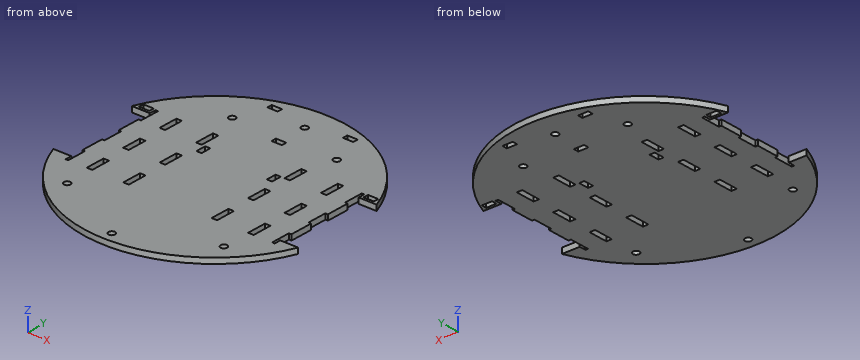
```python
from build123d import *

# Parameters (mm, degrees)
SKETCH1_R            = 127
BODY_DEPTH           = 5.334
SKETCH7_W            = 50.8
SKETCH7_H            = 88.9
WHEELCUTS_DEPTH      = 180.684310823
SKETCH4_W            = 2.4638
SKETCH4_H            = 19.05
SKETCH4_W_2          = 5.334
MOTORMOUNTS_DEPTH    = 175.099537782
SKETCH5_R            = 3.175
CASTOR_DEPTH         = 175.099537782
SKETCH6_R            = 3.175
BOLTHOLES_DEPTH      = 175.099537782
SKETCH3_W            = 10.000000066
SKETCH3_H            = 4.999999906
SKETCH3_W_2          = 5
SKETCH3_H_2          = 10
TAPESENSCUTOUT_DEPTH = 175.099537782


with BuildPart() as part:
    # Sketch1 → Body (new body)
    with BuildSketch(Plane.XY):
        Circle(SKETCH1_R)
    extrude(amount=BODY_DEPTH)

    # Sketch7 → WheelCuts (cut, through all)
    with BuildSketch(Plane.XY.offset(5.334)):
        with Locations((-127, 0)):
            Rectangle(SKETCH7_W, SKETCH7_H)
        with Locations((127, 0)):
            Rectangle(SKETCH7_W, SKETCH7_H)
    extrude(amount=-WHEELCUTS_DEPTH, mode=Mode.SUBTRACT)

    # Sketch4 → MotorMounts (cut, through all)
    with BuildSketch(Plane.XY.offset(5.334)):
        with Locations((-100.3681, 41.275)):
            Rectangle(SKETCH4_W, SKETCH4_H)
        with Locations((-100.3681, -41.275)):
            Rectangle(SKETCH4_W, SKETCH4_H)
        with Locations((-100.3681, 0)):
            Rectangle(SKETCH4_W, SKETCH4_H)
        with Locations((-78.469199932, -41.275)):
            Rectangle(SKETCH4_W_2, SKETCH4_H)
        with Locations((-78.469199932, 41.275)):
            Rectangle(SKETCH4_W_2, SKETCH4_H)
        with Locations((-78.469199932, 0)):
            Rectangle(SKETCH4_W_2, SKETCH4_H)
        with Locations((-42.966999918, -41.275)):
            Rectangle(SKETCH4_W_2, SKETCH4_H)
        with Locations((-42.966999918, 41.275)):
            Rectangle(SKETCH4_W_2, SKETCH4_H)
        with Locations((-42.966999918, 0)):
            Rectangle(SKETCH4_W_2, SKETCH4_H)
        with Locations((42.966999918, -41.275)):
            Rectangle(SKETCH4_W_2, SKETCH4_H)
        with Locations((42.966999918, 0)):
            Rectangle(SKETCH4_W_2, SKETCH4_H)
        with Locations((42.966999918, 41.275)):
            Rectangle(SKETCH4_W_2, SKETCH4_H)
        with Locations((78.469199932, -41.275)):
            Rectangle(SKETCH4_W_2, SKETCH4_H)
        with Locations((78.469199932, 0)):
            Rectangle(SKETCH4_W_2, SKETCH4_H)
        with Locations((78.469199932, 41.275)):
            Rectangle(SKETCH4_W_2, SKETCH4_H)
        with Locations((100.3681, -41.275)):
            Rectangle(SKETCH4_W, SKETCH4_H)
        with Locations((100.3681, 0)):
            Rectangle(SKETCH4_W, SKETCH4_H)
        with Locations((100.3681, 41.275)):
            Rectangle(SKETCH4_W, SKETCH4_H)
    extrude(amount=-MOTORMOUNTS_DEPTH, mode=Mode.SUBTRACT)

    # Sketch5 → Castor (cut, through all)
    with BuildSketch(Plane.XY.offset(5.334)):
        with Locations((0, -116.84)):
            Circle(SKETCH5_R)
        with Locations((0, 101.6)):
            Circle(SKETCH5_R)
    extrude(amount=-CASTOR_DEPTH, mode=Mode.SUBTRACT)

    # Sketch6 → BoltHoles (cut, through all)
    with BuildSketch(Plane.XY.offset(5.334)):
        with Locations((-76.2, -78.74)):
            Circle(SKETCH6_R)
        with Locations((-50.8, 78.74)):
            Circle(SKETCH6_R)
        with Locations(Location((76.2, -78.74, 0), (0, 0, 180))):
            Circle(SKETCH6_R)
        with Locations(Location((50.8, 78.74, 0), (0, 0, 180))):
            Circle(SKETCH6_R)
    extrude(amount=-BOLTHOLES_DEPTH, mode=Mode.SUBTRACT)

    # Sketch3 → TapeSensCutOut (cut, through all)
    with BuildSketch(Plane.XY.offset(5.334)):
        with Locations((-36.750000033, 110.449999953)):
            Rectangle(SKETCH3_W, SKETCH3_H)
        with Locations((-109.140000033, 49.489999953)):
            Rectangle(SKETCH3_W, SKETCH3_H)
        with Locations((36.750000033, 110.449999953)):
            Rectangle(SKETCH3_W, SKETCH3_H)
        with Locations((0, 72.349999953)):
            Rectangle(SKETCH3_W, SKETCH3_H)
        with Locations((109.140000033, 49.489999953)):
            Rectangle(SKETCH3_W, SKETCH3_H)
        with Locations((34.25, 26.75)):
            Rectangle(SKETCH3_W_2, SKETCH3_H_2)
        with Locations((-34.25, 26.75)):
            Rectangle(SKETCH3_W_2, SKETCH3_H_2)
    extrude(amount=-TAPESENSCUTOUT_DEPTH, mode=Mode.SUBTRACT)


solid = part.part
```
The listing builds one solid part. Answer for the finished solid, in the listing's coordinates (mm). Round coordinates to 2 decimals unless told otherwise and drop trailing zeros. Write each loop counter-clockwise with the first axis right and the second up, starting at its lowest first coordinate (ties: lowest second). Pieces come first, ordered by that corner, then holes. Notation, with made-up numbers: (25.5, 22.25) -> (62.5, 22.25) arc R26 cw to (62.5, 48.25) -> close; hole circle Ø9 at (-37.75, 68). An arc over 180 degrees is marked (long way). Use CSV: the item, a comma, the result in double quotes. Start each with the question number.
(1) Section B-B on x = 0 is taken. Give the vertices of the cut face in (y, z) (3 decimals), then the cut area to 3 significant figures.
(2) Consider L1, parallel to X at y = 35.5, z = 3.3; L2, parallel to Y at x = 0, z = 2 (3 decimals); L3, parallel to Y at x = 42.5, z = 4.5 (3 decimals). Determine where each line is inside the solid, lowest interval first. Write a range as from..to.
(3) Each of these flat-tipped pins is pushed along its axis until it touches: pin 1 (1 mm diameter, centred on y = -17.5, z = 0.5, fed in from +X); pin 2 (2.5 mm diameter, centred on y = -47.5, z = 3, fed in from +X); pin 3 (1.6 mm diameter, centred on x = 111, z = 3, fed in from -Y). Where does it stop, or does it pass through?
(4) Section C-C on x = 50.8 is taken. Give the vertices of the cut face in (y, z) (3 decimals).
(5) Section A-A on y = 101.6 is taken. Give the vertices of the cut face in (x, z) (3 decimals).
(6) Section D-D on z = 1.4 is taken. Count the separate pieces of the cut face and the enclosed holes in it, then the cut area to 3 significant figures.
A:
1,outline,"(-127, 0) -> (-120.015, 0) -> (-120.015, 5.334) -> (-127, 5.334) -> close; (-113.665, 0) -> (69.85, 0) -> (69.85, 5.334) -> (-113.665, 5.334) -> close; (74.85, 0) -> (98.425, 0) -> (98.425, 5.334) -> (74.85, 5.334) -> close; (104.775, 0) -> (127, 0) -> (127, 5.334) -> (104.775, 5.334) -> close"
1,area,"1,260 mm²"
2,L1,"x = -99.14..-81.14, -75.8..-45.63, -40.3..40.3, 45.63..75.8, 81.14..99.14"
2,L2,"y = -127..-120.015, -113.665..69.85, 74.85..98.425, 104.775..127"
2,L3,"y = -119.678..-50.8, -31.75..-9.525, 9.525..31.75, 50.8..119.678"
3,pin 1,"stops at x = 101.6"
3,pin 2,"stops at x = 118.28"
3,pin 3,"stops at y = -63.13"
4,outline,"(-116.397, 0) -> (75.565, 0) -> (75.565, 5.334) -> (-116.397, 5.334) -> close; (81.915, 0) -> (116.397, 0) -> (116.397, 5.334) -> (81.915, 5.334) -> close"
5,outline,"(-76.2, 0) -> (-3.175, 0) -> (-3.175, 5.334) -> (-76.2, 5.334) -> close; (3.175, 0) -> (76.2, 0) -> (76.2, 5.334) -> (3.175, 5.334) -> close"
6,separate pieces,"1"
6,enclosed holes,"25"
6,area,"44,600 mm²"
